Work out the finished part from the listing and answer in its coordinate system (mm). A direction names the side the tool comes from. Round coordinates to 2 decimals unless told otherwise and drop trailing zeros. Order: outer loops, then holes, each group sorted by start corner. A loop starts at its lowest first (then second) coordinate and runs counter-clockwise, first axis right, second up. Notation, with made-up numbers: (16.5, -11.5) - (28.5, -11.5) arc R23 cw to (28.5, -2.5) - close; hole circle Ø10 at (89.25, 44). An arc over 180 degrees is marked (long way). Put each result on its own line as item: value.
```python
from build123d import *

# Parameters (mm, degrees)
SKETCH1_W           = 50.8
SKETCH1_H           = 40.64
BOSS_EXTRUDE1_DEPTH = 1.7
SKETCH2_W           = 5
SKETCH2_H           = 26
BOSS_EXTRUDE2_DEPTH = 8.6
SKETCH3_W           = 5.5
SKETCH3_H           = 26
BOSS_EXTRUDE3_DEPTH = 8.6


with BuildPart() as part:
    # Sketch1 → Boss-Extrude1 (new body)
    with BuildSketch(Plane(origin=(0, 0, 0), x_dir=(1, 0, 0), z_dir=(0, 1, 0))):
        Rectangle(SKETCH1_W, SKETCH1_H)
    extrude(amount=BOSS_EXTRUDE1_DEPTH)

    # Sketch2 → Boss-Extrude2 (add)
    with BuildSketch(Plane.XZ):
        with Locations((-21.9, -6.32)):
            Rectangle(SKETCH2_W, SKETCH2_H)
    extrude(amount=BOSS_EXTRUDE2_DEPTH)

    # Sketch3 → Boss-Extrude3 (add)
    with BuildSketch(Plane.XZ):
        with Locations((20.93, -6.32)):
            Rectangle(SKETCH3_W, SKETCH3_H)
    extrude(amount=BOSS_EXTRUDE3_DEPTH)


solid = part.part
```
1) A cutting plane is placed at A-A on y = -2.75. Write down the section's boundary in (x, z), then the cut area to 3 significant figures.
Findings below:
outline: (-24.4, -19.32) - (-19.4, -19.32) - (-19.4, 6.68) - (-24.4, 6.68) - close; (18.18, -19.32) - (23.68, -19.32) - (23.68, 6.68) - (18.18, 6.68) - close
area: 273 mm2
2) A cutting plane is placed at B-B on x = 19.5. Write down the section's boundary in (y, z), then the cut area to 3 significant figures.
Findings below:
outline: (-8.6, -19.32) - (0, -19.32) - (0, -20.32) - (1.7, -20.32) - (1.7, 20.32) - (0, 20.32) - (0, 6.68) - (-8.6, 6.68) - close
area: 293 mm2
3) Straight lines are drawn through the part: L1, parallel to X at y = -8, z = -9; L2, parallel to Z at x = 21, y = -7.75; L3, parallel to Y at x = -12, z = -11. For each, find the intervals that lie inside material, in ascending order. Write a range as from..to.
Findings below:
L1: x = -24.4..-19.4, 18.18..23.68
L2: z = -19.32..6.68
L3: y = 0..1.7
4) A cutting plane is placed at D-D on x = 9. Write down the section's boundary in (y, z).
Findings below:
outline: (0, -20.32) - (1.7, -20.32) - (1.7, 20.32) - (0, 20.32) - close
5) For a pull along X with two mould halves and no side action, classify faces 1 (the flat face through (18.18, -4, -7)), 2 (the flat face through (21, -4, -19.32)), 3 (the flat face through (0, 0, 0)), 4 (the flat face through (25.4, 1, 0)) as pulls with the +X half, pulls with the -X half, needs draft (parallel to the pull), parting line crosses it, or undercut.
Findings below:
face 1: undercut
face 2: needs draft
face 3: undercut
face 4: pulls with the +X half
6) For faces 5 (the flat face through (23.68, -4, -7)), 6 (the flat face through (-22, -4, -19.32)), 7 (the flat face through (-24.4, -4, -7)), 8 (the flat face through (-19.4, -4, -7)), 9 (the flat face through (21, -4, 6.68)), determine the directions among +Z, -Z, +X, -X, +Y, -Y from which every point of the face is accessible in a straight line to the end or side of a thin tool.
Findings below:
face 5: +Z, -Z, +X, -Y
face 6: -Z, +X, -X, -Y
face 7: +Z, -Z, -X, -Y
face 8: +Z, -Z, -Y
face 9: +Z, +X, -X, -Y
7) A cutting plane is placed at C-C on z = -15.5. Write down the section's boundary in (x, y), then the cut area to 3 significant figures.
Findings below:
outline: (-25.4, 0) - (-24.4, 0) - (-24.4, -8.6) - (-19.4, -8.6) - (-19.4, 0) - (18.18, 0) - (18.18, -8.6) - (23.68, -8.6) - (23.68, 0) - (25.4, 0) - (25.4, 1.7) - (-25.4, 1.7) - close
area: 177 mm2
8) Given pin 1 Ø12 at (x, z) = (-5.5, 5) entering from -Y; pin 2 Ø2 at (y, z) = (-5, -7.5) entering from +X; pin 3 Ø2.5 at (y, z) = (-5.5, -10.5) entering from -X; pin 4 Ø6 at (x, y) = (15.5, -0.5) entering from -Z, each flat-ended and moving along its own axis, determine where each tip first touches the part or whether it passes through.
Findings below:
pin 1: stops at y = 0
pin 2: stops at x = 23.68
pin 3: stops at x = -24.4
pin 4: stops at z = -20.32
